Design review of the part built by this model. Coordinates are the model's own, in mm. A direction names the side the tool comes from. Give positions to 0.01 mm unless a question says otherwise; leave off trailing zeros. Order: outer loops, then holes, each group sorted by start corner. A loop starts at its lowest first (then second) coordinate and runs counter-clockwise, first axis right, second up. Notation, with made-up numbers: M 79.25,53 L 124.25,53 A17 cw 124.25,73 Z; hole C 4,5.5 d9. An arc over 180 degrees is marked long. Put each result on its own line as item: value. Start each with the question number.
from build123d import *

# Parameters (mm, degrees)
SKETCH_1_W      = 55
SKETCH_1_H      = 66
EXTRUDE_1_DEPTH = 30
FILLET_1_R      = 10
SKETCH_2_W      = 0.5
SKETCH_2_H      = 35.350562887
EXTRUDE_2_DEPTH = 0.5
SKETCH_2_4_W    = 0.5
SKETCH_2_4_H    = 35.350562887
EXTRUDE_4_DEPTH = 0.5
SKETCH_2_5_W    = 0.5
SKETCH_2_5_H    = 35.350562887
EXTRUDE_5_DEPTH = 0.5
SKETCH_2_6_W    = 0.5
SKETCH_2_6_H    = 35.350562887
EXTRUDE_6_DEPTH = 0.5
SKETCH_2_7_W    = 1.5
SKETCH_2_7_H    = 35.350562887
EXTRUDE_7_DEPTH = 0.5


with BuildPart() as part:
    # 草图1 → 凸台-拉伸1 (new body)
    with BuildSketch(Plane.XY):
        Rectangle(SKETCH_1_W, SKETCH_1_H)
    extrude(amount=EXTRUDE_1_DEPTH)

    # 圆角1
    fillet_1_edges = [part.edges().sort_by_distance(p)[0] for p in [
        (-27.5, 0, 30),
        (0, -33, 30),
        (27.5, 0, 30),
        (0, -33, 0),
        (-27.5, 0, 0),
        (0, 33, 0),
        (27.5, 0, 0),
        (27.5, -33, 15),
        (-27.5, -33, 15),
        (-27.5, 33, 15),
        (27.5, 33, 15),
        (0, 33, 30),
    ]]
    fillet(fillet_1_edges, radius=FILLET_1_R)

    # 草图2 → 凸台-拉伸2 (add)
    with BuildSketch(Plane.ZY.offset(17.5)):
        with Locations((13.5, 50.675281444)):
            Rectangle(SKETCH_2_W, SKETCH_2_H)
    extrude(amount=-EXTRUDE_2_DEPTH)

    # 草图2<4> → 凸台-拉伸4 (add)
    with BuildSketch(Plane.ZY.offset(17.5)):
        with Locations((14, 50.675281444)):
            Rectangle(SKETCH_2_4_W, SKETCH_2_4_H)
    extrude(amount=-EXTRUDE_4_DEPTH)

    # 草图2<5> → 凸台-拉伸5 (add)
    with BuildSketch(Plane.ZY.offset(17.5)):
        with Locations((15, 50.675281444)):
            Rectangle(SKETCH_2_5_W, SKETCH_2_5_H)
    extrude(amount=-EXTRUDE_5_DEPTH)

    # 草图2<6> → 凸台-拉伸6 (add)
    with BuildSketch(Plane.ZY.offset(17.5)):
        with Locations((14.5, 50.675281444)):
            Rectangle(SKETCH_2_6_W, SKETCH_2_6_H)
    extrude(amount=-EXTRUDE_6_DEPTH)

    # 草图2<7> → 凸台-拉伸7 (add)
    with BuildSketch(Plane.ZY.offset(17.5)):
        with Locations((16, 50.675281444)):
            Rectangle(SKETCH_2_7_W, SKETCH_2_7_H)
    extrude(amount=-EXTRUDE_7_DEPTH)


solid = part.part
1. Machinability: for faces 1 (the cylindrical face through (0.25, 30.15, 3.01)), 2 (the flat face through (-17.5, 51, 15)), 3 (the flat face through (-17, 51, 15)), which of the approach directions +Z, -Z, +X, -X, +Y, -Y give a long, thin tool a straight path to every point of the face, cutting with its end or side? Answer none if there is none.
2. Consider section B-B on x = 23.5. Give the boundary of the cut face in (y, z), then the cut area to 3 significant figures.
3. Insertion check: pin 1 (1.8 mm diameter, centred on y = 58.5, z = 14, fed in from -X); pin 2 (3 mm diameter, centred on x = 6.5, z = 17, fed in from +Y); pin 3 (1.5 mm diameter, centred on x = 16, z = 9, fed in from -Y). Each pin has a flat end and moves straight along its axis. Give the tip position at first contact, or say it passes through.
4. To check wall thickness, follow probe 1 along X at (y, z) = (36, 14.25); probe 2 along Y at (x, z) = (1.5, 9.5); probe 3 along Y at (x, z) = (19, 13.75). State the ranges of each line that lie inside material, in increasing order.
5. Consider section A-A on y = -8. Give the boundary of the cut face in (x, z), then the cut area to 3 significant figures.
6. Consider section C-C on y = 41.5. Give the boundary of the cut face in (x, z).
Returned:
1. face 1: -Z, +X, -X, +Y
1. face 2: +Z, -Z, -X, +Y
1. face 3: +Z, -Z, +X, +Y
2. outline: M -31,10 A8 ccw -23,2 L 23,2 A8 ccw 31,10 L 31,20 A8 ccw 23,28 L -23,28 A8 ccw -31,20 Z
2. area: 1,560 mm2
3. pin 1: stops at x = -17.5
3. pin 2: stops at y = 33
3. pin 3: stops at y = -33
4. probe 1: x = -17.5 to -17
4. probe 2: y = -32.99 to 32.99
4. probe 3: y = -32.89 to 32.89
5. outline: M -27.5,10 A10 ccw -17.5,0 L 17.5,0 A10 ccw 27.5,10 L 27.5,20 A10 ccw 17.5,30 L -17.5,30 A10 ccw -27.5,20 Z
5. area: 1,560 mm2
6. outline: M -17.5,13.25 L -17,13.25 L -17,16.75 L -17.5,16.75 Z
